Geometry check sheet. Reference: the model listing, model coordinates, mm. Round coordinates to 2 decimals unless told otherwise and drop trailing zeros. Write each loop counter-clockwise with the first axis right and the second up, starting at its lowest first coordinate (ties: lowest second). Pieces come first, ordered by that corner, then holes. Notation, with made-up numbers: (40.25, 49) -> (63.25, 49) arc R33 cw to (63.25, 88) -> close; hole circle Ø4 at (77, -3.5). An arc over 180 degrees is marked (long way). Put each result on its own line as item: value. Start each with the question number.
from build123d import *

# Parameters (mm, degrees)
RESSALTO_EXTRUS_O1_DEPTH = 1.9
ESBO_O2_R                = 14.25
CORTE_EXTRUS_O1_DEPTH    = 1.9
FILETE1_R                = 13
FILETE2_R                = 35


with BuildPart() as part:
    # Esboço1 → Ressalto-extrusão1 (new body)
    with BuildSketch(Plane.XY):
        Polygon((-160, 70), (0, 120), (170, 120), (170, 0), (0, 0), (0, -30), (-160, -30), align=None)
    extrude(amount=RESSALTO_EXTRUS_O1_DEPTH)

    # Esboço2 → Corte-extrusão1 (cut)
    with BuildSketch(Plane.XY.offset(1.9)):
        with Locations((-50, -10)):
            Circle(ESBO_O2_R)
        with Locations((-130, 30)):
            Circle(ESBO_O2_R)
    extrude(amount=-CORTE_EXTRUS_O1_DEPTH, mode=Mode.SUBTRACT)

    # Filete1
    filete1_edges = [part.edges().sort_by_distance(p)[0] for p in [
        (0, 0, 0.95),
    ]]
    fillet(filete1_edges, radius=FILETE1_R)

    # Filete2
    filete2_edges = [part.edges().sort_by_distance(p)[0] for p in [
        (-160, 70, 0.95),
        (0, 120, 0.95),
        (170, 120, 0.95),
    ]]
    fillet(filete2_edges, radius=FILETE2_R)


solid = part.part
(1) Go/stop test with flat-tipped pins: pin 1 Ø17 at (x, y) = (-50, -10) entering from +Z; pin 2 Ø0.6 at (x, z) = (68, 1.5) entering from -Y; pin 3 Ø1 at (y, z) = (-20, 1) entering from +X. Record where each tip stops, or that it passes through.
(2) Material ranges on L1, parallel to X at y = -7, z = 1.8; L2, parallel to X at y = 31, z = 0.4; L3, parallel to Y at x = -50, z = 1.25 (3 decimals), recorded low to high. Write a range as from..to.
(3) Mould release check, pull along X, two halves, no side actions. Record for faces 1 (the flat face through (-71.181, 97.756, 0.937)), 2 (the cylindrical face through (-60.503, -0.369, 0.963)), 3 (the cylindrical face through (-116.837, 24.542, 0.963)), 4 (the cylindrical face through (160.019, 109.475, 0.963)): +X half, -X half, draft (parallel to the pull), parting line (faces both ways), or undercut.
(4) Sectioned sample at B-B (x = -130). Record the cut outline in (y, z) (3 decimals), and give its area (3 significant figures).
(5) Sectioned sample at C-C (x = 28.5). Record the cut outline in (y, z), and give its area (3 significant figures).
(6) Sectioned sample at A-A (y = 30). Record the cut outline in (x, z).
(7) Sectioned sample at D-D (y = 71.5). Record the cut outline in (x, z).
Found:
1. pin 1: through
1. pin 2: y = 0
1. pin 3: x = 0
2. L1: -160..-63.93, -36.07..1.47
2. L2: -160..-144.21, -115.79..170
2. L3: -30..-24.25, 4.25..104.375
3. face 1: -X half
3. face 2: undercut
3. face 3: undercut
3. face 4: +X half
4. outline: (-30, 0) -> (15.75, 0) -> (15.75, 1.9) -> (-30, 1.9) -> close; (44.25, 0) -> (79.375, 0) -> (79.375, 1.9) -> (44.25, 1.9) -> close
4. area: 154 mm2
5. outline: (0, 0) -> (120, 0) -> (120, 1.9) -> (0, 1.9) -> close
5. area: 228 mm2
6. outline: (-160, 0) -> (-144.25, 0) -> (-144.25, 1.9) -> (-160, 1.9) -> close; (-115.75, 0) -> (170, 0) -> (170, 1.9) -> (-115.75, 1.9) -> close
7. outline: (-146.99, 0) -> (170, 0) -> (170, 1.9) -> (-146.99, 1.9) -> close
